```python
from build123d import *

# Parameters (mm, degrees)
F0_W     = 835.025
F0_H     = 762
F1_DEPTH = 19.05
F2_W     = 6.35
F2_H     = 165.1
F3_DEPTH = 19.051
F2_H_2   = 298.45
F4_DEPTH = 12.7
F5_R     = 4.0132
F5_R_2   = 6.35
F6_DEPTH = 25.4


with BuildPart() as f1:
    # F0 (on Top) → F1 (new body)
    with BuildSketch(Plane.XY):
        Rectangle(F0_W, F0_H)
    extrude(amount=F1_DEPTH)

    # F2 (on face) → F3 (cut, through all)
    with BuildSketch(Plane.XY.offset(19.05)):
        with Locations((-420.6875, 0)):
            Rectangle(F2_W, F2_H)
        with Locations((-414.3375, 0)):
            Rectangle(F2_W, F2_H)
        with BuildLine():
            Line((-401.6375, 82.55), (-411.1625, 82.55))
            Line((-411.1625, 82.55), (-411.1625, -82.55))
            Line((-411.1625, -82.55), (-401.6375, -82.55))
            ThreePointArc((-401.6375, -82.55), (-394.9023079092, -79.7601920908), (-392.1125, -73.025))
            Line((-392.1125, -73.025), (-392.1125, 73.025))
            ThreePointArc((-392.1125, 73.025), (-394.9023079092, 79.7601920908), (-401.6375, 82.55))
        make_face()
        with BuildLine():
            Line((411.1625, -82.55), (411.1625, 82.55))
            Line((411.1625, 82.55), (401.6375, 82.55))
            ThreePointArc((401.6375, 82.55), (394.9023079092, 79.7601920908), (392.1125, 73.025))
            Line((392.1125, 73.025), (392.1125, -73.025))
            ThreePointArc((392.1125, -73.025), (394.9023079092, -79.7601920908), (401.6375, -82.55))
            Line((401.6375, -82.55), (411.1625, -82.55))
        make_face()
        with Locations((420.6875, 0)):
            Rectangle(F2_W, F2_H)
        with Locations((414.3375, 0)):
            Rectangle(F2_W, F2_H)
    extrude(amount=-F3_DEPTH, mode=Mode.SUBTRACT)

    # F2 (on face) → F4 (cut)
    with BuildSketch(Plane.XY.offset(19.05)):
        with Locations((-414.3375, 231.775)):
            Rectangle(F2_W, F2_H_2)
        with Locations((-414.3375, -231.775)):
            Rectangle(F2_W, F2_H_2)
        with Locations((414.3375, 231.775)):
            Rectangle(F2_W, F2_H_2)
        with Locations((414.3375, -231.775)):
            Rectangle(F2_W, F2_H_2)
        with BuildLine():
            ThreePointArc((202.40625, -373.85625), (197.3548559319, -375.9486059319), (195.2625, -381))
            Line((195.2625, -381), (322.2625, -381))
            ThreePointArc((322.2625, -381), (320.1701440681, -375.9486059319), (315.11875, -373.85625))
            Line((315.11875, -373.85625), (202.40625, -373.85625))
        make_face()
        with BuildLine():
            ThreePointArc((-315.11875, -373.85625), (-320.1701440681, -375.9486059319), (-322.2625, -381))
            Line((-322.2625, -381), (-195.2625, -381))
            ThreePointArc((-195.2625, -381), (-197.3548559319, -375.9486059319), (-202.40625, -373.85625))
            Line((-202.40625, -373.85625), (-315.11875, -373.85625))
        make_face()
    extrude(amount=-F4_DEPTH, mode=Mode.SUBTRACT)

    # F5 (on face) → F6 (cut)
    with BuildSketch(Plane.XY.offset(19.05)):
        with Locations((-368.3, 63.5)):
            Circle(F5_R)
        with Locations((-368.3, 88.9)):
            Circle(F5_R)
        with Locations((-368.3, 114.3)):
            Circle(F5_R)
        with Locations((-368.3, 139.7)):
            Circle(F5_R)
        with Locations((-368.3, 165.1)):
            Circle(F5_R)
        with Locations((-368.3, 190.5)):
            Circle(F5_R)
        with Locations((-368.3, 215.9)):
            Circle(F5_R)
        with Locations((-368.3, 241.3)):
            Circle(F5_R)
        with Locations((-368.3, 266.7)):
            Circle(F5_R)
        with Locations((-368.3, 292.1)):
            Circle(F5_R)
        with Locations((-368.3, 317.5)):
            Circle(F5_R)
        with Locations((-368.3, 342.9)):
            Circle(F5_R)
        with Locations((-368.3, 368.3)):
            Circle(F5_R)
        with Locations((368.3, 317.5)):
            Circle(F5_R)
        with Locations((368.3, 292.1)):
            Circle(F5_R)
        with Locations((368.3, 266.7)):
            Circle(F5_R)
        with Locations((368.3, 241.3)):
            Circle(F5_R)
        with Locations((368.3, 215.9)):
            Circle(F5_R)
        with Locations((368.3, 190.5)):
            Circle(F5_R)
        with Locations((368.3, 165.1)):
            Circle(F5_R)
        with Locations((368.3, 139.7)):
            Circle(F5_R)
        with Locations((368.3, 114.3)):
            Circle(F5_R)
        with Locations((368.3, 368.3)):
            Circle(F5_R)
        with Locations((368.3, 342.9)):
            Circle(F5_R)
        with Locations((368.3, 88.9)):
            Circle(F5_R)
        with Locations((368.3, 63.5)):
            Circle(F5_R)
        with BuildLine():
            Line((-368.3, -63.5), (-364.2868, -63.5))
            ThreePointArc((-364.2868, -63.5), (-371.1377609343, -60.6622390657), (-368.3, -67.5132))
            Line((-368.3, -67.5132), (-368.3, -63.5))
        make_face()
        with BuildLine():
            ThreePointArc((-364.2868, -88.9), (-365.4622390657, -86.0622390657), (-368.3, -84.8868))
            ThreePointArc((-368.3, -84.8868), (-371.1377609343, -91.7377609343), (-364.2868, -88.9))
        make_face()
        with BuildLine():
            ThreePointArc((-368.3, -67.5132), (-365.4622390657, -66.3377609343), (-364.2868, -63.5))
            Line((-364.2868, -63.5), (-368.3, -63.5))
            Line((-368.3, -63.5), (-368.3, -67.5132))
        make_face()
        with Locations((-368.3, -317.5)):
            Circle(F5_R)
        with Locations((-368.3, -292.1)):
            Circle(F5_R)
        with Locations((-368.3, -266.7)):
            Circle(F5_R)
        with Locations((-368.3, -241.3)):
            Circle(F5_R)
        with Locations((-368.3, -215.9)):
            Circle(F5_R)
        with Locations((368.3, -292.1)):
            Circle(F5_R)
        with Locations((-368.3, -190.5)):
            Circle(F5_R)
        with Locations((-368.3, -165.1)):
            Circle(F5_R)
        with Locations((-368.3, -139.7)):
            Circle(F5_R)
        with Locations((368.3, -190.5)):
            Circle(F5_R)
        with Locations((-368.3, -114.3)):
            Circle(F5_R)
        with Locations((368.3, -368.3)):
            Circle(F5_R)
        with Locations((368.3, -266.7)):
            Circle(F5_R)
        with Locations((368.3, -342.9)):
            Circle(F5_R)
        with Locations((368.3, -63.5)):
            Circle(F5_R)
        with Locations((368.3, -241.3)):
            Circle(F5_R)
        with Locations((368.3, -165.1)):
            Circle(F5_R)
        with Locations((368.3, -317.5)):
            Circle(F5_R)
        with Locations((368.3, -88.9)):
            Circle(F5_R)
        with Locations((368.3, -139.7)):
            Circle(F5_R)
        with Locations((368.3, -215.9)):
            Circle(F5_R)
        with Locations((-368.3, -342.9)):
            Circle(F5_R)
        with Locations((-368.3, -368.3)):
            Circle(F5_R)
        with Locations((368.3, -114.3)):
            Circle(F5_R)
        with Locations((-368.3, 0)):
            Circle(F5_R_2)
        with Locations((368.3, 0)):
            Circle(F5_R_2)
    extrude(amount=-F6_DEPTH, mode=Mode.SUBTRACT)


solid = f1.part
```
Geometry: final body of the model. Coordinates: model frame, mm. A direction names the side the tool comes from. Coordinates: 2 decimals unless noted, no trailing zeros. Use a Markdown table: item, result. Add a question column.
(1) Pin query (flat end, axial travel): pin 1 Ø4 at (y, z) = (-252, 10) entering from -X; pin 2 Ø4 at (y, z) = (245, 14) entering from +X. Return the tip coordinate at first contact, or that it passes through.
(2) Mould query, pull axis Y, two halves, no side actions, for faces 3 (the flat face through (-6, 5, 19.05)), 4 (the flat face through (-6, -381, 9)), 5 (the flat face through (-6, 381, 9)), 6 (the flat face through (392.112, 1, 10)). Classes: pulls with the +Y half, pulls with the -Y half, needs draft (parallel to the pull), parting line crosses it, or undercut.
(3) Section query A-A, the plane z = 11.25. State how many separate pieces and enclosed holes the cut face has, plus the area to 3 significant figures.
(4) Access query for faces 1 (the flat face through (-6, 5, 0)), 2 (the flat face through (-392.112, -1, 10)). Directions: +Z, -Z, +X, -X, +Y, -Y. A direction counts if a zero-diameter tool reaches every point of the face in a straight line with its end or side. Return the directions, or none.
(5) Line query: line 1 along X through (y, z) = (-266.7, 13.25); line 2 along X through (y, z) = (339.5, 1.5); line 3 along X through (y, z) = (-224, 17.75). Output: solid intervals per line, ascending.
Answer:
| question | item | result |
|---|---|---|
| 1 | pin 1 | stops at x = -411.16 |
| 1 | pin 2 | stops at x = 411.16 |
| 2 | face 3 | needs draft |
| 2 | face 4 | pulls with the -Y half |
| 2 | face 5 | pulls with the +Y half |
| 2 | face 6 | undercut |
| 3 | separate pieces | 1 |
| 3 | enclosed holes | 54 |
| 3 | area | 616,000 mm^2 |
| 4 | face 1 | -Z, +X, -X, +Y, -Y |
| 4 | face 2 | +Z, -Z, -X |
| 5 | line 1 | x = -411.16 to -372.31, -364.29 to 364.29, 372.31 to 411.16 |
| 5 | line 2 | x = -417.51 to -370.43, -366.17 to 366.17, 370.43 to 417.51 |
| 5 | line 3 | x = -411.16 to 411.16 |
